```python
from build123d import *

# Parameters (mm, degrees)
SKETCH1_W           = 40.6
SKETCH1_H           = 21
BOSS_EXTRUDE1_DEPTH = 1.5
SKETCH2_W           = 3.76
SKETCH2_H           = 3
BOSS_EXTRUDE3_DEPTH = 1.1
SKETCH3_R           = 0.25
CUT_EXTRUDE1_DEPTH  = 0.5
FILLET3_R           = 0.5
SKETCH4_R           = 0.65
BOSS_EXTRUDE4_DEPTH = 0.25


with BuildPart() as part:
    # Sketch1 → Boss-Extrude1 (new body)
    with BuildSketch(Plane.XY):
        with Locations((20.3, 10.5)):
            Rectangle(SKETCH1_W, SKETCH1_H)
    extrude(amount=BOSS_EXTRUDE1_DEPTH)

    # Sketch2 → Boss-Extrude3 (add)
    with BuildSketch(Plane(origin=(0, 0, 0), x_dir=(-1, 0, 0), z_dir=(0, 0, -1))):
        with Locations((-8.38, 13.31)):
            Rectangle(SKETCH2_W, SKETCH2_H)
    extrude(amount=BOSS_EXTRUDE3_DEPTH)

    # Sketch3 → Cut-Extrude1 (cut)
    with BuildSketch(Plane(origin=(0, 0, -1.1), x_dir=(-1, 0, 0), z_dir=(0, 0, -1))):
        with Locations((-9.08, 13.31)):
            Circle(SKETCH3_R)
    extrude(amount=-CUT_EXTRUDE1_DEPTH, mode=Mode.SUBTRACT)

    # Fillet3
    fillet3_edges = [part.edges().sort_by_distance(p)[0] for p in [
        (6.5, 13.31, -1.1),
        (8.38, 14.81, -1.1),
        (10.26, 13.31, -1.1),
        (8.38, 11.81, -1.1),
    ]]
    fillet(fillet3_edges, radius=FILLET3_R)

    # Sketch4 → Boss-Extrude4 (add)
    with BuildSketch(Plane(origin=(0, 0, 0), x_dir=(-1, 0, 0), z_dir=(0, 0, -1))):
        with Locations((-18.925, 3.72)):
            Circle(SKETCH4_R)
        with Locations((-20.675, 3.72)):
            Circle(SKETCH4_R)
        with Locations((-20.675, 5.47)):
            Circle(SKETCH4_R)
        with Locations((-20.675, 7.22)):
            Circle(SKETCH4_R)
        with Locations((-18.925, 5.47)):
            Circle(SKETCH4_R)
        with Locations((-18.925, 7.22)):
            Circle(SKETCH4_R)
    extrude(amount=BOSS_EXTRUDE4_DEPTH)


solid = part.part
```
CAD build for the part. Positions are in the model's coordinates, mm. Coordinates: 2 decimals unless noted, no trailing zeros. Write each loop counter-clockwise with the first axis right and the second up, starting at its lowest first coordinate (ties: lowest second). Pieces come first, ordered by that corner, then holes. Notation, with made-up numbers: (-33, -40) -> (-10, -40) arc R25 cw to (-10, -24) -> close; hole circle Ø8 at (-32.5, 57). An arc over 180 degrees is marked (long way). Return JSON: item names as keys, results as strings. Group by question number.
Q1. Cut at A-A, the plane y = 5.47. Give the cut face in (x, z) (3 decimals), then the cut area to 4 significant figures.
Q2. Cut at B-B, the plane x = 5.5. Give the cut face in (y, z), then the cut area to 3 significant figures.
Q3. Drill centre lines: line 1 (Y direction, x = 9.08, z = -0.65); line 2 (Z direction, x = 25.5, y = 7); line 3 (Y direction, x = 9.08, z = -0.85). Where is each one in solid material? Low to high.
Q4. Cut at C-C, the plane y = 17. Give the cut face in (x, z).
Q5. Flat gauge pins, fed straight in: pin 1 (10 mm diameter, centred on x = 25.5, y = 10, fed in from -Z); pin 2 (6.5 mm diameter, centred on x = 10.5, y = 6, fed in from -Z). Where does each tip first touch, or does it go through?
Returned:
{
 "1": {"outline": "(0, 0) -> (18.275, 0) -> (18.275, -0.25) -> (19.575, -0.25) -> (19.575, 0) -> (20.025, 0) -> (20.025, -0.25) -> (21.325, -0.25) -> (21.325, 0) -> (40.6, 0) -> (40.6, 1.5) -> (0, 1.5) -> close", "area": "61.55 mm2"},
 "2": {"outline": "(0, 0) -> (21, 0) -> (21, 1.5) -> (0, 1.5) -> close", "area": "31.5 mm2"},
 "3": {"line 1": "y = 11.81 to 13.06, 13.56 to 14.81", "line 2": "z = 0 to 1.5", "line 3": "y = 11.88 to 13.06, 13.56 to 14.74"},
 "4": {"outline": "(0, 0) -> (40.6, 0) -> (40.6, 1.5) -> (0, 1.5) -> close"},
 "5": {"pin 1": "stops at z = -0.25", "pin 2": "stops at z = 0"}
}
